```python
from build123d import *

# Parameters (mm, degrees)
F0_R      = 12.7
F1_DEPTH  = 25.4
F3_DEPTH  = 10.16
F4_DEPTH  = 10.16
F6_DEPTH  = 20.066
F8_DEPTH  = 19.812
F9_R      = 5.46143
F11_DEPTH = 25.4
F10_R     = 5.353375
F12_DEPTH = 25.4


with BuildPart() as f1:
    # F0 (on Front) → F1 (new body)
    with BuildSketch(Plane.XZ):
        with BuildLine():
            ThreePointArc((-52.411983, 19.05), (-38.941599, 13.470384), (-33.361983, 0))
            ThreePointArc((-33.361983, 0), (-38.941599, -13.470384), (-52.411983, -19.05))
            Line((-52.411983, -19.05), (52.411983, -19.05))
            ThreePointArc((52.411983, -19.05), (33.361983, 0), (52.411983, 19.05))
            Line((52.411983, 19.05), (-52.411983, 19.05))
        make_face()
        with BuildLine():
            ThreePointArc((-52.411983, -19.05), (-38.941599, -13.470384), (-33.361983, 0))
            ThreePointArc((-33.361983, 0), (-38.941599, 13.470384), (-52.411983, 19.05))
            ThreePointArc((-52.411983, 19.05), (-71.461983, 0), (-52.411983, -19.05))
        make_face()
        with Locations((-52.411983, 0)):
            Circle(F0_R, mode=Mode.SUBTRACT)
        with BuildLine():
            ThreePointArc((71.461983, 0), (65.882367, 13.470384), (52.411983, 19.05))
            ThreePointArc((52.411983, 19.05), (33.361983, 0), (52.411983, -19.05))
            ThreePointArc((52.411983, -19.05), (65.882367, -13.470384), (71.461983, 0))
        make_face()
        with Locations((52.411983, 0)):
            Circle(F0_R, mode=Mode.SUBTRACT)
    extrude(amount=F1_DEPTH)

    # F2 (on Top) → F3 (join)
    with BuildSketch(Plane.XY):
        with BuildLine():
            Line((-38.1, 0), (0, 0))
            Line((0, 0), (38.1, 0))
            Line((38.1, 0), (38.1, 35.410588))
            Line((38.1, 35.410588), (18.377647, 35.410588))
            ThreePointArc((18.377647, 35.410588), (0, 21.363075), (-18.377647, 35.410588))
            Line((-18.377647, 35.410588), (-38.1, 35.410588))
            Line((-38.1, 35.410588), (-38.1, 0))
        make_face()
    extrude(amount=F3_DEPTH)

    # F3_face (on face) → F4 (join)
    with BuildSketch(Plane(origin=(0, 15.751851, 0), x_dir=(1, 0, 0), z_dir=(0, 0, -1))):
        with BuildLine():
            Line((38.1, 15.751851), (-38.1, 15.751851))
            Line((-38.1, 15.751851), (-38.1, -19.658738))
            Line((-38.1, -19.658738), (-18.377647, -19.658738))
            ThreePointArc((-18.377647, -19.658738), (0, -5.611224), (18.377647, -19.658738))
            Line((18.377647, -19.658738), (38.1, -19.658738))
            Line((38.1, -19.658738), (38.1, 15.751851))
        make_face()
    extrude(amount=F4_DEPTH)

    # F5 (on face) → F6 (join)
    with BuildSketch(Plane(origin=(-38.1, 0, 0), x_dir=(0, -1, 0), z_dir=(-1, 0, 0))):
        with BuildLine():
            Line((-35.410588, -10.16), (-35.410588, 10.16))
            ThreePointArc((-35.410588, 10.16), (-45.570588, 0), (-35.410588, -10.16))
        make_face()
    extrude(amount=-F6_DEPTH)

    # F7 (on face) → F8 (join)
    with BuildSketch(Plane.YZ.offset(38.1)):
        with BuildLine():
            Line((35.410588, 10.16), (35.410588, -10.16))
            ThreePointArc((35.410588, -10.16), (45.570588, 0), (35.410588, 10.16))
        make_face()
    extrude(amount=-F8_DEPTH)

    # F9 (on face) → F11 (cut)
    with BuildSketch(Plane(origin=(-38.1, 0, 0), x_dir=(0, -1, 0), z_dir=(-1, 0, 0))):
        with Locations((-35.410588, 0)):
            Circle(F9_R)
    extrude(amount=-F11_DEPTH, mode=Mode.SUBTRACT)

    # F10 (on face) → F12 (cut)
    with BuildSketch(Plane.YZ.offset(38.1)):
        with Locations((35.410588, 0)):
            Circle(F10_R)
    extrude(amount=-F12_DEPTH, mode=Mode.SUBTRACT)


solid = f1.part
```
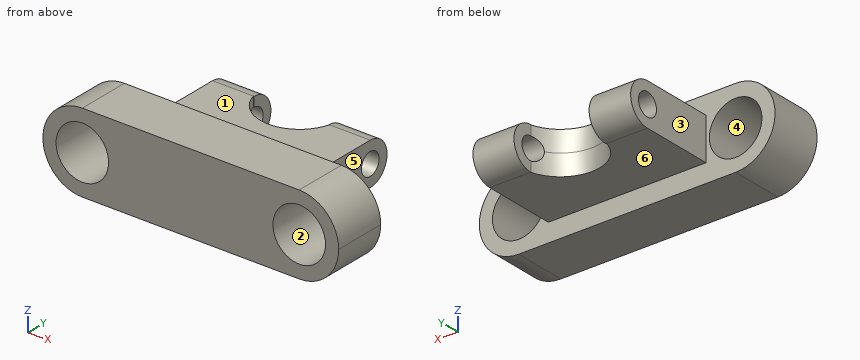
Verification items for the finished model (mm, model axes). Face numbers are marked on the shaded views. A direction names the side the tool comes from. Round coordinates to 2 decimals unless told otherwise and drop trailing zeros. Write each loop counter-clockwise with the first axis right and the second up, starting at its lowest first coordinate (ties: lowest second). Pieces come first, ordered by that corner, then holes. Notation, with made-up numbers: (-37, 42) -> (-12, 42) arc R15 cw to (-12, 55) -> close; hole circle Ø9 at (-36, 81). An arc over 180 degrees is marked (long way). Write each question's results on one line, items separated by ' | '. Start each with the question number.
1. Depth check by flat-ended pin: P1, Ø16.5, axis at y = 33, z = -1, coming from the +X side; P2, Ø12, axis at x = 55.5, z = -15, coming from the +Y side; P3, Ø12, axis at x = 22, y = 30.5, coming from the -Z side. Enter the tip coordinate at first touch or a pass-through.
2. Draft check along X on the marked faces 4, 5 and 6. Enter one of: +X half, -X half, draft (parallel to the pull), parting line (faces both ways), or undercut.
3. Cross-section at A-A (x = 33). Enter the section's corners in (y, z), then the cut area to 3 significant figures.
4. Cross-section at D-D (y = 39). Enter the section's corners in (x, z), then the cut area to 3 significant figures.
5. Set-up check for the marked faces 1, 2 and 3: record each of +Z, -Z, +X, -X, +Y, -Y from which the full face is reachable in a straight line by a thin tool's end or side.
6. Cross-section at B-B (y = 23.5). Enter the section's corners in (x, z), then the cut area to 3 significant figures.
7. Material ranges on probe 1 along Y at (x, z) = (22.75, 0); probe 2 along Y at (x, z) = (-21.75, 0); probe 3 along Z at (x, y) = (-1, 18), recorded low to high. Write a range as from..to.
8. Cross-section at C-C (z = 3). Enter the section's corners in (x, y).
Solutions:
1) P1: stops at x = 38.1 | P2: stops at y = 0 | P3: stops at z = -10.16
2) face 4: undercut | face 5: +X half | face 6: draft
3) outline: (-25.4, -19.05) -> (0, -19.05) -> (0, -10.16) -> (35.41, -10.16) arc R10.16 ccw to (35.41, 10.16) -> (0, 10.16) -> (0, 19.05) -> (-25.4, 19.05) -> close; hole circle Ø10.71 at (35.41, 0) | area: 1,760 mm2
4) outline: (-38.1, -9.5) -> (-18.03, -9.5) -> (-18.03, -4.12) -> (-38.1, -4.12) -> close; (-38.1, 4.12) -> (-18.03, 4.12) -> (-18.03, 9.5) -> (-38.1, 9.5) -> close; (18.29, -9.5) -> (38.1, -9.5) -> (38.1, -3.97) -> (18.29, -3.97) -> close; (18.29, 3.97) -> (38.1, 3.97) -> (38.1, 9.5) -> (18.29, 9.5) -> close | area: 435 mm2
5) face 1: +Z, +X, -X, +Y | face 2: +Y, -Y | face 3: +Z, -Z, -X, +Y
6) outline: (-38.1, -10.16) -> (-8.77, -10.16) -> (-8.77, 10.16) -> (-38.1, 10.16) -> close; (8.77, -10.16) -> (38.1, -10.16) -> (38.1, 10.16) -> (8.77, 10.16) -> close | area: 1,190 mm2
7) probe 1: y = -25.4..30.06, 40.76..45.57 | probe 2: y = -25.4..29.95, 40.87..45.57 | probe 3: z = -10.16..10.16
8) outline: (-71.22, -25.4) -> (-64.75, -25.4) -> (-64.75, 0) -> (-71.22, 0) -> close; (-40.07, -25.4) -> (40.07, -25.4) -> (40.07, 0) -> (38.1, 0) -> (38.1, 30.98) -> (16.55, 30.98) arc R19.05 cw to (-16.47, 30.85) -> (-38.1, 30.85) -> (-38.1, 0) -> (-40.07, 0) -> close; (-38.1, 39.97) -> (-18.03, 39.97) -> (-18.03, 45.12) -> (-38.1, 45.12) -> close; (18.29, 39.84) -> (38.1, 39.84) -> (38.1, 45.12) -> (18.29, 45.12) -> close; (64.75, -25.4) -> (71.22, -25.4) -> (71.22, 0) -> (64.75, 0) -> close
